Autodesk Inventor part; units mm, degrees
ref_plane "Work Plane1" through (0, 4.7283, -22.9522) normal (-1, 0, 0) x (0, -0.8411785, 0.5407576)
ref_plane "Work Plane2" through (178, -56.0619, -70.2985) normal (1, 0, 0) x (0, 0.8411785, -0.5407576)
ref_plane "Work Plane3" through (22, -31.0502, -8.6656) normal (0, -0.7712334, 0.6365525) x (1, 0, 0)
ref_plane "Work Plane1" through (0, 4.7283, -22.9522) normal (-1, 0, 0) x (0, -0.8411785, 0.5407576)
sketch "Sketch1" plane through (0, 4.7283, -22.9522) normal (-1, 0, 0) x (0, -0.8411785, 0.5407576)
  line L0 (61.5, -12.25) -> (61.5, -16.75)
  line L1 (61.5, -16.75) -> (65.5, -16.75)
  line L2 (65.5, -16.75) -> (65.5, -20.25)
  line L3 (65.5, -20.25) -> (79.5, -20.25)
  line L4 (79.5, -20.25) -> (65.5, -11.25)
  line L5 (65.5, -11.25) -> (65.5, -12.25)
  line L6 (65.5, -12.25) -> (61.5, -12.25)
  line L7 (16.3889, 16.75) -> (16.3889, 18.75)
  line L8 (14.7421, 12.75) -> (16.3889, 18.75)
  line L9 (63.3493, -12.25) -> (12.0798, 20.7089)
  line L10 (16.3889, 16.75) -> (16.3889, 17.9388)
  arc A0 (-57.551, -16.75) -> (-61.5, -12.801) centre (-58.75, -14) ccw
  arc A1 (-34.301, -16.75) -> (-36.699, -16.75) centre (-35.5, -14) ccw
  line L11 (61.5, -12.25) -> (16.3889, 16.75)
  line L12 (16.3889, 13.75) -> (-61.5, 13.75)
  line L13 (-61.5, 13.75) -> (-61.5, -12.801)
  line L14 (-61.5, 13.75) -> (-61.5, -12.801)
  arc A2 (-57.551, -16.75) -> (-61.5, -12.801) centre (-58.75, -14) ccw
  line L15 (-57.551, -16.75) -> (-36.699, -16.75)
  arc A3 (-34.301, -16.75) -> (-36.699, -16.75) centre (-35.5, -14) ccw
  line L16 (-34.301, -16.75) -> (61.5, -16.75)
  line L17 (61.5, -16.75) -> (61.5, -12.25)
  line L18 (21.0556, 13.75) -> (-61.5, 13.75)
  line L19 (-57.551, -16.75) -> (-36.699, -16.75)
  line L20 (-34.301, -16.75) -> (61.5, -16.75)
  line L21 (61.5, -16.75) -> (61.5, -12.25)
  line L22 (61.5, -12.25) -> (21.0556, 13.75)
  point P0 (16.3889, 17.9388)
  point P1 (15.5655, 15.75)
  point P2 (16.3889, 17.9388)
  point P3 (16.1996, 18.0605)
  dimension "d14" = 1
  dimension "d15" = 2
ref_plane "Work Plane2" through (178, -56.0619, -70.2985) normal (1, 0, 0) x (0, 0.8411785, -0.5407576)
extrude "Extrusion1" add sketch "Sketch1" against normal up to surface (178 mm away) contours L11 L7 L9 L6
sketch "Sketch2" plane through (0, -55.184, 1) normal (0, 0, 1) x (1, 0, 0)
  circle A0 centre (3, 16.4427) radius 2.5
  circle A1 centre (3, 35.7569) radius 2.5
  line L0 (0, 2.3333) -> (0, 55.184)
  line L1 (0, 2.3333) -> (3, 2.3333)
  line L2 (6, 50.414) -> (6, 9.4662)
  line L3 (0, 50.414) -> (6, 50.414)
  circle A2 centre (175, 21.9904) radius 2.5
  circle A3 centre (175, 41.3047) radius 2.5
  line L4 (178, 2.3333) -> (178, 55.9618)
  line L5 (178, 55.9618) -> (172, 55.9618)
  line L6 (172, 55.9618) -> (172, 2.3333)
  line L7 (178, 2.3333) -> (172, 2.3333)
  line L8 (3, 9.4662) -> (3, 2.3333)
  line L9 (3, 9.4662) -> (6, 9.4662)
  point P0 (3, 35.7569)
  point P1 (3, 16.4427)
hole "Hole1" at (3, -19.4271, 1) at (3, -38.7413, 1) at (175, -33.1936, 1) at (175, -13.8793, 1) direction (0, 0, -1) diameter 3.6 end through all countersink diameter 7 countersink angle 90
ref_plane "Work Plane3" through (22, -31.0502, -8.6656) normal (0, -0.7712334, 0.6365525) x (1, 0, 0)
sketch "Sketch3" plane through (22, -31.0502, -8.6656) normal (0, -0.7712334, 0.6365525) x (1, 0, 0)
  line L0 (-9.9215, 5.3729) -> (-9.9215, -5.5323)
  spline S0 degree 3 poles (-9.9215, -5.5323) (-9.9222, -5.6561) (-9.8204, -5.8999) (-9.5772, -6.0011) (-9.4534, -6.0004) knots 0 0 0 0 0.5 1 1 1 1
  line L1 (-9.4534, -6.0004) -> (19.4534, -6.0004)
  spline S1 degree 3 poles (19.4534, -6.0004) (19.5775, -6.0011) (19.8219, -5.8989) (19.9222, -5.6548) (19.9215, -5.5307) knots 0 0 0 0 0.5 1 1 1 1
  line L2 (19.9215, -5.5307) -> (19.9215, 5.3744)
  spline S2 degree 3 poles (19.9215, 5.3744) (19.9222, 5.4985) (19.82, 5.743) (19.5758, 5.8433) (19.4518, 5.8426) knots 0 0 0 0 0.5 1 1 1 1
  line L3 (19.4518, 5.8426) -> (-9.4534, 5.8426)
  spline S3 degree 3 poles (-9.4534, 5.8426) (-9.5775, 5.8433) (-9.8219, 5.7411) (-9.9222, 5.4969) (-9.9215, 5.3729) knots 0 0 0 0 0.5 1 1 1 1
  circle A0 centre (-8.3791, -4.458) radius 0.5
  circle A1 centre (-8.3791, 4.3001) radius 0.5
  circle A2 centre (18.3791, 4.3001) radius 0.5
  circle A3 centre (18.3791, -4.458) radius 0.5
  arc A4 (5.2617, -1.5301) -> (5.1811, -1.6008) centre (5.2771, -1.6289) ccw
  arc A5 (5.1811, 1.4429) -> (5.1811, -1.6008) centre (0, -0.0789) ccw
  arc A6 (5.1811, 1.4429) -> (5.2617, 1.3723) centre (5.2771, 1.4711) ccw
  arc A7 (5.2617, 1.3723) -> (5.3414, 1.4401) centre (5.2463, 1.4711) ccw
  arc A8 (5.3414, -1.5979) -> (5.3414, 1.4401) centre (10, -0.0789) ccw
  arc A9 (5.3414, -1.5979) -> (5.2617, -1.5301) centre (5.2463, -1.6289) ccw
  line L4 (143.9215, 5.3729) -> (143.9215, -5.5323)
  spline S4 degree 3 poles (143.4534, 5.8426) (143.5775, 5.8433) (143.8219, 5.7411) (143.9222, 5.4969) (143.9215, 5.3729) knots 0 0 0 0 0.5 1 1 1 1
  line L5 (114.5482, 5.8426) -> (143.4534, 5.8426)
  spline S5 degree 3 poles (114.0785, 5.3744) (114.0778, 5.4985) (114.18, 5.743) (114.4242, 5.8433) (114.5482, 5.8426) knots 0 0 0 0 0.5 1 1 1 1
  line L6 (114.0785, -5.5307) -> (114.0785, 5.3744)
  spline S6 degree 3 poles (114.5466, -6.0004) (114.4225, -6.0011) (114.1781, -5.8989) (114.0778, -5.6548) (114.0785, -5.5307) knots 0 0 0 0 0.5 1 1 1 1
  line L7 (143.4534, -6.0004) -> (114.5466, -6.0004)
  spline S7 degree 3 poles (143.9215, -5.5323) (143.9222, -5.6561) (143.8204, -5.8999) (143.5772, -6.0011) (143.4534, -6.0004) knots 0 0 0 0 0.5 1 1 1 1
  circle A10 centre (142.3791, -4.458) radius 0.5
  circle A11 centre (142.3791, 4.3001) radius 0.5
  circle A12 centre (115.6209, 4.3001) radius 0.5
  circle A13 centre (115.6209, -4.458) radius 0.5
  arc A14 (128.8189, -1.6008) -> (128.7383, -1.5301) centre (128.7229, -1.6289) ccw
  arc A15 (128.7383, -1.5301) -> (128.6586, -1.5979) centre (128.7537, -1.6289) ccw
  arc A16 (128.6586, 1.4401) -> (128.6586, -1.5979) centre (124, -0.0789) ccw
  arc A17 (128.6586, 1.4401) -> (128.7383, 1.3723) centre (128.7537, 1.4711) ccw
  arc A18 (128.7383, 1.3723) -> (128.8189, 1.4429) centre (128.7229, 1.4711) ccw
  arc A19 (128.8189, -1.6008) -> (128.8189, 1.4429) centre (134, -0.0789) ccw
  circle A20 centre (10, -0.0789) radius 5.4
  circle A21 centre (124, -0.0789) radius 5.4
  line L8 (0, 5.3211) -> (10, 5.3211)
  line L9 (10, -5.4789) -> (0, -5.4789)
  line L10 (124, 5.3211) -> (134, 5.3211)
  line L11 (134, -5.4789) -> (124, -5.4789)
  point P0 (-22, 26.4483)
  point P1 (14.6373, -1.6617)
  point P2 (5, 1.9607)
  point P3 (5.3627, -1.6617)
  point P4 (5, -2.1185)
  point P5 (7.5029, -4.2949)
  point P6 (3.3743, -4.2949)
  point P7 (5.2923, -1.5401)
  dimension "d9" = 10.8
  dimension "d10" = 10.8
extrude "Extrusion2" cut sketch "Sketch3" along normal blind 78.25 contours A9 A8 A7 A6 A5 A20 A4 | A4 A5 A20 A6 A7 A8 A9 | A5 A20 | A19 A21 A18 A17 A16 A15 A14 | A14 A15 A16 A17 A18 A19 A21 | A21 A19 | A19 L11 A21 | A19 A21 L10
properties part number "front" material "Aluminum 6061"
The model under review builds one solid part; all positions refer to its coordinate system, in mm. A direction names the side the tool comes from. Coordinates: 2 decimals unless noted, no trailing zeros. Order: outer loops, then holes, each group sorted by start corner. A loop starts at its lowest first (then second) coordinate and runs counter-clockwise, first axis right, second up. Notation, with made-up numbers: (66, 9.25) -> (109, 9.25) arc R11 cw to (109, 18.25) -> close; hole circle Ø8 at (-33, -10.5). An arc over 180 degrees is marked (long way). Answer in a Markdown table with one row per item. Add a question column.
Item 1: To check wall thickness, follow probe 1 along Y at (x, z) = (36.5, 0.45); probe 2 along X at (y, z) = (-49.5, 0.4) (3 decimals); probe 3 along X at (y, z) = (-32, 0.3). State the ranges of each line that lie inside material, in increasing order.
Item 2: Machinability: for faces 3 (the cylindrical face through (161.4, -42.2, 0.5)), 4 (the conical face through (172.39, -32.614, 0.174)), which of the approach directions +Z, -Z, +X, -X, +Y, -Y give a long, thin tool a straight path to every point of the face, cutting with its end or side? Answer none if there is none.
Item 3: We need section B-B on z = 0.2. Give the number of separate pieces and of enclosed holes in the cut face, plus the area to 3 significant figures.
Item 4: We need section A-A on x = 3. Write out the cut boundary in (y, z), plus the area to 3 significant figures.
Item 5: We need section C-C on x = 90.5. Write out the cut boundary in (y, z), plus the area to 3 significant figures.
Item 6: Mouldability with a two-part tool opening along X and no side actions: class faces 1 (the flat face through (88, -27, 0)), 2 (the cylindrical face through (140.6, -42.3, 0.4)) as +X half, -X half, draft (parallel to the pull), parting line (faces both ways), or undercut.
Final values:
| question | item | result |
|---|---|---|
| 1 | probe 1 | y = -54.33 to -46.91, -37.53 to 0.29 |
| 1 | probe 2 | x = 0 to 19.295, 24.705 to 29.295, 34.705 to 143.295, 158.705 to 178 |
| 1 | probe 3 | x = 0 to 172.47, 177.53 to 178 |
| 2 | face 3 | none |
| 2 | face 4 | +Z |
| 3 | separate pieces | 1 |
| 3 | enclosed holes | 6 |
| 3 | area | 8,930 mm2 |
| 4 | outline | (-55.18, 1) -> (-53.63, 0) -> (-41.24, 0) -> (-42.24, 1) -> close; (-36.24, 0) -> (-21.93, 0) -> (-22.93, 1) -> (-35.24, 1) -> close; (-16.93, 0) -> (0, 0) -> (0.64, 1) -> (-15.93, 1) -> close |
| 4 | area | 42.7 mm2 |
| 5 | outline | (-55.18, 1) -> (-53.63, 0) -> (0, 0) -> (0.64, 1) -> close |
| 5 | area | 54.7 mm2 |
| 6 | face 1 | draft |
| 6 | face 2 | undercut |
